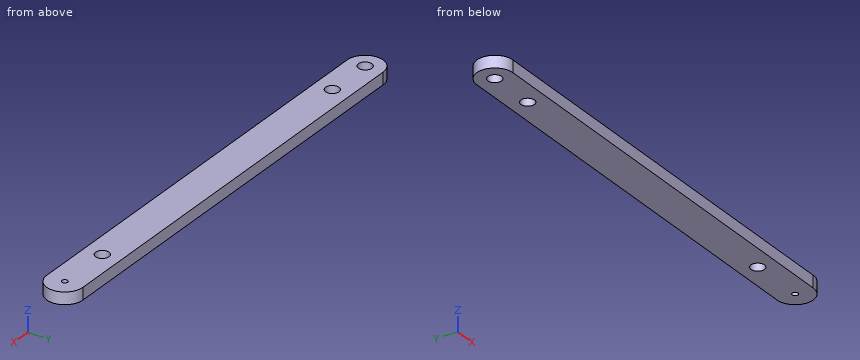
from build123d import *

# Parameters (mm, degrees)
SKETCH1_R                       = 0.762
BOSS_EXTRUDE1_DEPTH             = 3.175
F_9_64_0_14063_DIAMETER_HOLE1_D = 3.572002
F_9_64_0_14063_DIAMETER_HOLE2_D = 3.572002
F_9_64_0_14063_DIAMETER_HOLE3_D = 3.572002


with BuildPart() as part:
    # Sketch1 → Boss-Extrude1 (new body)
    with BuildSketch(Plane.XY):
        with BuildLine():
            Line((-10.922, -4.7625), (-127, -4.7625))
            ThreePointArc((-127, -4.7625), (-131.7625, 0), (-127, 4.7625))
            Line((-127, 4.7625), (-25.4, 4.7625))
            Line((-25.4, 4.7625), (-10.922, 4.7625))
            ThreePointArc((-10.922, 4.7625), (-6.1595, 0), (-10.922, -4.7625))
        make_face()
        with Locations((-25.4, 0)):
            Circle(SKETCH1_R, mode=Mode.SUBTRACT)
        with Locations((-10.922, 0)):
            Circle(SKETCH1_R, mode=Mode.SUBTRACT)
    extrude(amount=BOSS_EXTRUDE1_DEPTH)

    # 9/64 (0.14063) Diameter Hole1 (through all)
    with Locations(Plane.XY.offset(3.175)):
        with Locations((0, 0), (-127, 0)):
            Hole(F_9_64_0_14063_DIAMETER_HOLE1_D / 2)

    # 9/64 (0.14063) Diameter Hole2 (through all)
    with Locations(Plane.XY.offset(3.175)):
        with Locations((-114.3, 0)):
            Hole(F_9_64_0_14063_DIAMETER_HOLE2_D / 2)

    # 9/64 (0.14063) Diameter Hole3 (through all)
    with Locations(Plane.XY.offset(3.175)):
        with Locations((-25.4, 0)):
            Hole(F_9_64_0_14063_DIAMETER_HOLE3_D / 2)


solid = part.part
Work out the finished part from the listing and answer in its coordinate system (mm). Round coordinates to 2 decimals unless told otherwise and drop trailing zeros. Order: outer loops, then holes, each group sorted by start corner. A loop starts at its lowest first (then second) coordinate and runs counter-clockwise, first axis right, second up. Notation, with made-up numbers: M 6.25,-21 L 57.25,-21 A29 ccw 57.25,17 Z; hole C -17,44.25 d8. An arc over 180 degrees is marked long. Put each result on its own line as item: value. Start each with the question number.
Q1. Section A-A, the plane z = 2.45 is taken. Write down the section's boundary in (x, y) (1 decimal).
Q2. Section C-C, the plane y = -3.75 is taken. Write down the section's boundary in (x, z) (3 decimals), and give its area (3 significant figures).
Q3. Straight lines are drawn through the part: L1, parallel to Y at x = -114.3, z = 1.05; L2, parallel to X at y = 1.5, z = 3; L3, parallel to X at y = -0.25, z = 1.2. For each, find the intervals that lie inside material, in ascending order. Write a range as [from, to].
Q4. Section B-B, the plane x = -114.3 is taken. Write down the section's boundary in (y, z) (1 decimal).
Q5. A flat-ended cylindrical pin translates along its axis: pin 1 (1 mm diameter, centred on y = -2.5, z = 2, fed in from -X). Find the tip coordinate at first contact, or state that the pin passes through.
Findings below:
1. outline: M -127,-4.8 L -10.9,-4.8 A4.8 ccw -10.9,4.8 L -127,4.8 A4.8 ccw Z; hole C -127,0 d3.6; hole C -114.3,0 d3.6; hole C -25.4,0 d3.6; hole C -10.9,0 d1.5
2. outline: M -129.936,0 L -7.986,0 L -7.986,3.175 L -129.936,3.175 Z
2. area: 387 mm^2
3. L1: y = [-4.76, -1.79], [1.79, 4.76]
3. L2: x = [-131.52, -127.97], [-126.03, -115.27], [-113.33, -26.37], [-24.43, -6.4]
3. L3: x = [-131.76, -128.77], [-125.23, -116.07], [-112.53, -27.17], [-23.63, -11.64], [-10.2, -6.17]
4. outline: M -4.8,0 L -1.8,0 L -1.8,3.2 L -4.8,3.2 Z; M 1.8,0 L 4.8,0 L 4.8,3.2 L 1.8,3.2 Z
5. pin 1: stops at x = -131.32
